The drawing under review shows one solid part. Ordinate dimensions are in mm from its lowest x, y, z. A direction names the side the tool comes from. Coordinates: 2 decimals unless noted, no trailing zeros. Write each loop counter-clockwise with the first axis right and the second up, starting at its lowest first coordinate (ties: lowest second). Pieces come first, ordered by that corner, then holes. Notation, with made-up numbers: (62.5, -36) - (75.5, -36) arc R30 ccw to (75.5, -14) - close; hole circle Ø4 at (75.25, -14). An arc over 180 degrees is marked (long way). Use a Markdown table: item, result.
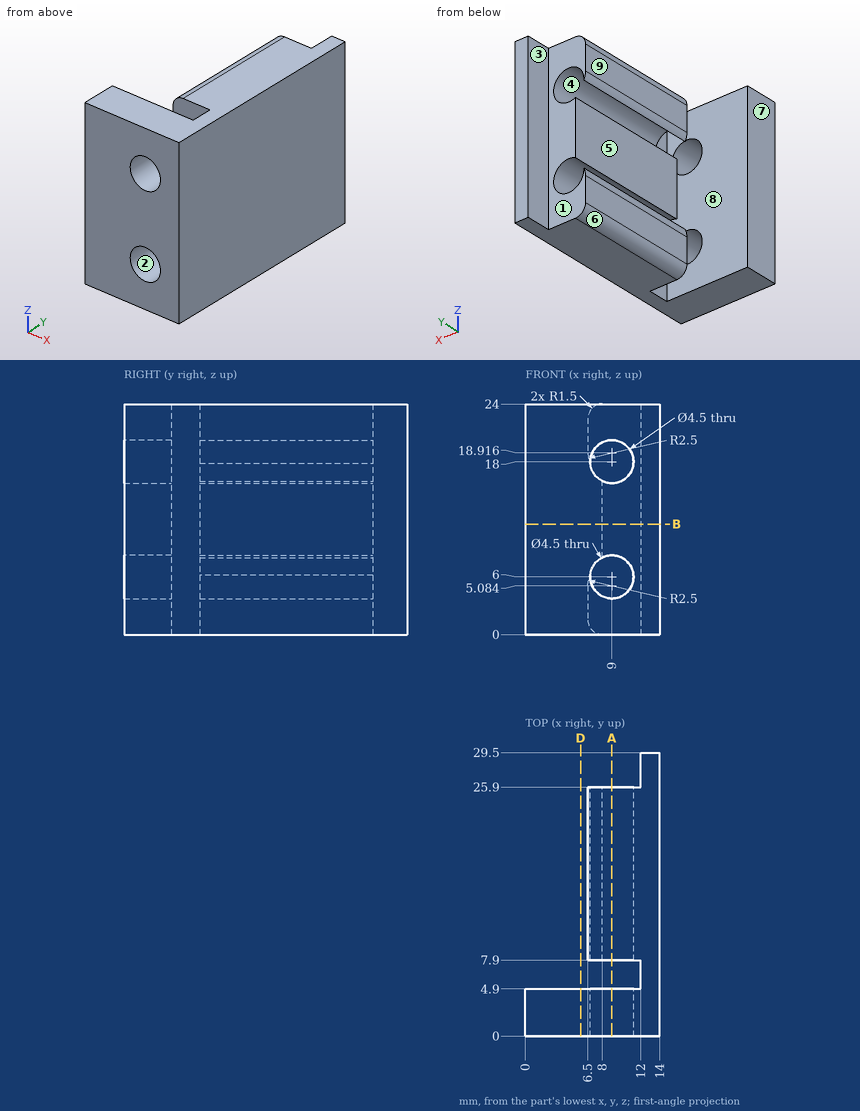
(1) For L1, parallel to X at y = 1.95, z = 18; L2, parallel to Y at x = 9.5, z = 10; L3, parallel to Z at x = 9, y = 16.5, list the stretches that pass through material, from the lowest coordinate up. Write a range as from..to.
Determined:
| item | result |
|---|---|
| L1 | 0..6.75, 11.25..14 |
| L2 | 0..4.9, 7.9..25.9 |
| L3 | 0..3.75, 8.25..15.75, 20.25..24 |
(2) Take a section at D-D on x = 5.75. Write out the cut boundary in (y, z).
Determined:
| item | result |
|---|---|
| outline | (0, 0) - (4.9, 0) - (4.9, 24) - (0, 24) - close |
(3) Take a section at B-B on z = 11.5. Write out the cut boundary in (x, y), and give its area (3 significant figures).
Determined:
| item | result |
|---|---|
| outline | (0, 0) - (14, 0) - (14, 29.5) - (12, 29.5) - (12, 25.9) - (8, 25.9) - (8, 7.9) - (12, 7.9) - (12, 4.9) - (0, 4.9) - close |
| area | 190 mm2 |
(4) Machinability: for the marked faces 5, 6, 7, 8 and 9, which of the approach directions +Z, -Z, +X, -X, +Y, -Y give a long, thin tool a straight path to every point of the face, cutting with its end or side? Answer none if there is none.
Determined:
| item | result |
|---|---|
| face 5 | -X, +Y |
| face 6 | -Z, -X, +Y |
| face 7 | +Z, -Z, -X, +Y, -Y |
| face 8 | +Z, -Z, -X |
| face 9 | +Z, -Z, -X, +Y |
(5) Take a section at A-A on x = 9. Write out the cut boundary in (y, z).
Determined:
| item | result |
|---|---|
| outline | (0, 0) - (4.9, 0) - (4.9, 3.75) - (0, 3.75) - close; (0, 8.25) - (4.9, 8.25) - (4.9, 15.75) - (0, 15.75) - close; (0, 20.25) - (4.9, 20.25) - (4.9, 24) - (0, 24) - close; (7.9, 0) - (25.9, 0) - (25.9, 3.75) - (7.9, 3.75) - close; (7.9, 8.25) - (25.9, 8.25) - (25.9, 15.75) - (7.9, 15.75) - close; (7.9, 20.25) - (25.9, 20.25) - (25.9, 24) - (7.9, 24) - close |
(6) For pin 1 (4 mm diameter, centred on y = 28, z = 6.5, fed in from -X); pin 2 (1.6 mm diameter, centred on x = 8, z = 9, fed in from +Y); pin 3 (1.1 mm diameter, centred on y = 18.5, z = 20, fed in from -X), all flat-tipped, find the tip position at first contact; note any pin that passes through.
Determined:
| item | result |
|---|---|
| pin 1 | x = 12 |
| pin 2 | y = 25.9 |
| pin 3 | x = 6.5 |
(7) Draft analysis for pull direction X (two halves, no side actions). For the marked faces 1, 2, 3 and 4, state which applies: +X half, -X half, draft (parallel to the pull), parting line (faces both ways), or undercut.
Determined:
| item | result |
|---|---|
| face 1 | draft |
| face 2 | undercut |
| face 3 | -X half |
| face 4 | undercut |
